Geometry: see drawing. Coordinates: mm, zero at the bounding-box minimum. A direction names the side the tool comes from. Coordinates: 2 decimals unless noted, no trailing zeros. Loops run counter-clockwise (first coordinate to the right, second up) from the corner with the lowest first, then second, coordinate; pieces in that order, holes last. Notation, with made-up numbers: (12.5, 89) -> (70.5, 89) arc R24 cw to (70.5, 123) -> close; hole circle Ø3 at (-9, -15.75). An arc over 180 degrees is marked (long way). Put each result on its own line as item: value. Start each with the question number.
1) Material intervals for L1, parallel to Z at x = 13.4, y = 0.2 (3 decimals); L2, parallel to Z at x = 18.8, y = 5.44; L3, parallel to Y at x = 20.1, z = 10.46, sorted ascending.
2) Cut plane B-B (y = 5.44). Return the cut outline in (x, z), plus the area to 3 significant figures.
3) Cut plane A-A (x = 13.4). Return the cut outline in (y, z) (3 decimals).
4) Contact query for flat-ended pins moving along their axis: P1, Ø1.1, axis at y = 0.5, z = 3, coming from the +X side (3 decimals); P2, Ø4.5, axis at y = 4.5, z = 10.5, coming from the +X side; P3, Ø5.5, axis at y = 5.44, z = 10.46, coming from the -X side; P4, Ø1.4, axis at x = 13, z = 4, coming from the +Y side. Output: stop coordinate, or through.
5) Cut plane C-C (z = 28.5). Return the cut outline in (x, y) (3 decimals), plus the area to 3 significant figures.
6) Cut plane D-D (z = 10.46). Return the cut outline in (x, y).
7) Pull-direction query (Y, two-part tool) for the marked faces 3, 4 and 5; classes: pulls with the +Y half, pulls with the -Y half, needs draft (parallel to the pull), parting line crosses it, or undercut.
8) Set-up query: the marked faces 1 and 2. Return all of +Z, -Z, +X, -X, +Y, -Y with unobstructed straight access to the full face (end or side cutting, diameter ignored); none if empty.
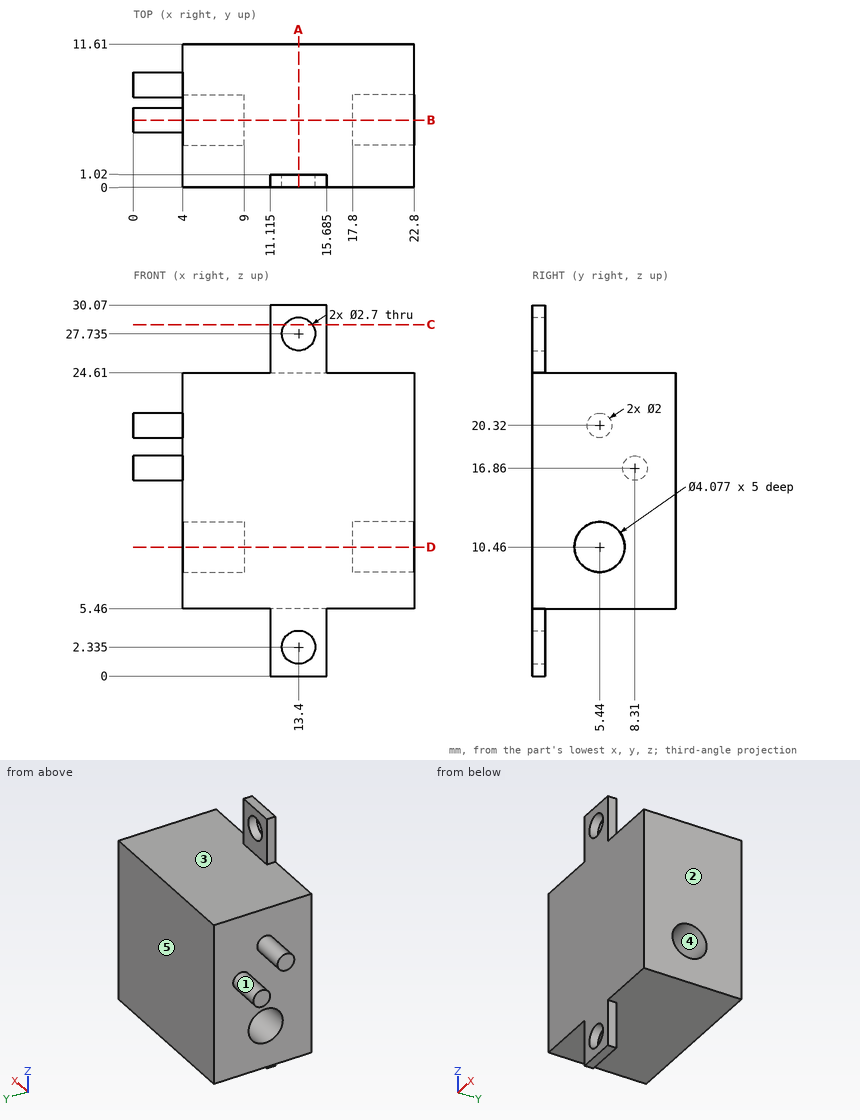
Results found:
1. L1: z = 0 to 0.985, 3.685 to 26.385, 29.085 to 30.07
1. L2: z = 5.46 to 8.42, 12.5 to 24.61
1. L3: y = 0 to 3.4, 7.48 to 11.61
2. outline: (0, 19.32) -> (4, 19.32) -> (4, 12.5) -> (9, 12.5) -> (9, 8.42) -> (4, 8.42) -> (4, 5.46) -> (22.8, 5.46) -> (22.8, 8.42) -> (17.8, 8.42) -> (17.8, 12.5) -> (22.8, 12.5) -> (22.8, 24.61) -> (4, 24.61) -> (4, 21.32) -> (0, 21.32) -> close
2. area: 327 mm2
3. outline: (0, 0) -> (1.02, 0) -> (1.02, 0.985) -> (0, 0.985) -> close; (0, 3.685) -> (1.02, 3.685) -> (1.02, 5.46) -> (11.61, 5.46) -> (11.61, 24.61) -> (1.02, 24.61) -> (1.02, 26.385) -> (0, 26.385) -> close; (0, 29.085) -> (1.02, 29.085) -> (1.02, 30.07) -> (0, 30.07) -> close
4. P1: stops at x = 15.685
4. P2: stops at x = 22.8
4. P3: stops at x = 4
4. P4: stops at y = 1.02
5. outline: (11.115, 0) -> (12.288, 0) -> (12.288, 1.02) -> (11.115, 1.02) -> close; (14.512, 0) -> (15.685, 0) -> (15.685, 1.02) -> (14.512, 1.02) -> close
5. area: 2.39 mm2
6. outline: (4, 0) -> (22.8, 0) -> (22.8, 3.4) -> (17.8, 3.4) -> (17.8, 7.48) -> (22.8, 7.48) -> (22.8, 11.61) -> (4, 11.61) -> (4, 7.48) -> (9, 7.48) -> (9, 3.4) -> (4, 3.4) -> close
7. face 3: needs draft
7. face 4: undercut
7. face 5: pulls with the +Y half
8. face 1: -X
8. face 2: +Z, -Z, +X, +Y, -Y
